The model under review builds one solid part; all positions refer to its coordinate system, in mm. A direction names the side the tool comes from. Round coordinates to 2 decimals unless told otherwise and drop trailing zeros. Loops run counter-clockwise (first coordinate to the right, second up) from the corner with the lowest first, then second, coordinate; pieces in that order, holes last. Notation, with made-up numbers: (-18, 43.5) -> (16, 43.5) arc R21 cw to (16, 81.5) -> close; hole circle Ø1 at (88.5, 79). An arc over 180 degrees is marked (long way). Use a Markdown table: item, result. Add a question column.
1) Consider section B-B on x = 0. Give the boundary of the cut face in (y, z), plus the area to 3 significant figures.
2) Consider section C-C on y = 2.5. Give the boundary of the cut face in (x, z).
3) Insertion check: pin 1 (2 mm diameter, centred on x = 0.5, z = -1, fed in from -Y); pin 2 (1 mm diameter, centred on y = 3.5, z = -0.5, fed in from -X); pin 3 (1 mm diameter, centred on x = -0.5, y = 2.5, fed in from -Z). Each pin has a flat end and moves straight along its axis. Give the tip position at first contact, or say it passes through.
4) Wall thickness on probe 1 along Z at (x, y) = (0.05, 3); probe 2 along Y at (x, z) = (-1.3, 1.1); probe 3 along X at (y, z) = (2.5, 0.65): over which ranges is each line inside the solid? List them lowest first.
5) For faces 1 (the cylindrical face through (-1.617, 0.507, 0.67)), 2 (the cylindrical face through (1.5, 2.52, -0.07)), list the 3-axis set-ups (+Z, -Z, +X, -X, +Y, -Y) from which the entire face can be reached by the end or side of a thin tool; tool diameter is ignored.
6) Consider section D-D on x = -0.7. Give the boundary of the cut face in (y, z).
7) Consider section A-A on z = 0. Give the boundary of the cut face in (x, y) (3 decimals), plus the area to 3 significant figures.
from build123d import *

# Parameters (mm, degrees)
SKETCH2_R           = 0.25
BOSS_EXTRUDE1_DEPTH = 3


with BuildPart() as part:
    # Sketch1 → Revolve1 (revolve)
    with BuildSketch(Plane.XY):
        with BuildLine():
            Line((0, 0), (-1.75, 0))
            Line((-1.75, 0), (-1.75, 1))
            Line((-1.75, 1), (-1.5, 1))
            Line((-1.5, 1), (-1.5, 4))
            ThreePointArc((-1.5, 4), (-1.060660172, 5.060660172), (0, 5.5))
            Line((0, 5.5), (0, 0))
        make_face()
    revolve(axis=Axis((0, 5.5, 0), (0, -1, 0)))

    # Sketch2 → Boss-Extrude1 (add)
    with BuildSketch(Plane.XZ):
        with Locations((-1.375, 0)):
            Circle(SKETCH2_R)
        with Locations((1.375, 0)):
            Circle(SKETCH2_R)
    extrude(amount=BOSS_EXTRUDE1_DEPTH)


solid = part.part
Result set:
| question | item | result |
|---|---|---|
| 1 | outline | (0, -1.75) -> (1, -1.75) -> (1, -1.5) -> (4, -1.5) arc R1.5 ccw to (4, 1.5) -> (1, 1.5) -> (1, 1.75) -> (0, 1.75) -> close |
| 1 | area | 16.0 mm2 |
| 2 | outline | circle Ø3 at (0, 0) |
| 3 | pin 1 | y = 0 |
| 3 | pin 2 | x = -1.5 |
| 3 | pin 3 | z = -1.5 |
| 4 | probe 1 | -1.5 to 1.5 |
| 4 | probe 2 | 0 to 1 |
| 4 | probe 3 | -1.35 to 1.35 |
| 5 | face 1 | +Y, -Y |
| 5 | face 2 | +Y |
| 6 | outline | (0, -1.6) -> (1, -1.6) -> (1, -1.33) -> (4, -1.33) arc R1.33 ccw to (4, 1.33) -> (1, 1.33) -> (1, 1.6) -> (0, 1.6) -> close |
| 7 | outline | (-1.75, 0) -> (-1.625, 0) -> (-1.625, -3) -> (-1.125, -3) -> (-1.125, 0) -> (1.125, 0) -> (1.125, -3) -> (1.625, -3) -> (1.625, 0) -> (1.75, 0) -> (1.75, 1) -> (1.5, 1) -> (1.5, 4) arc R1.5 ccw to (-1.5, 4) -> (-1.5, 1) -> (-1.75, 1) -> close |
| 7 | area | 19.0 mm2 |
